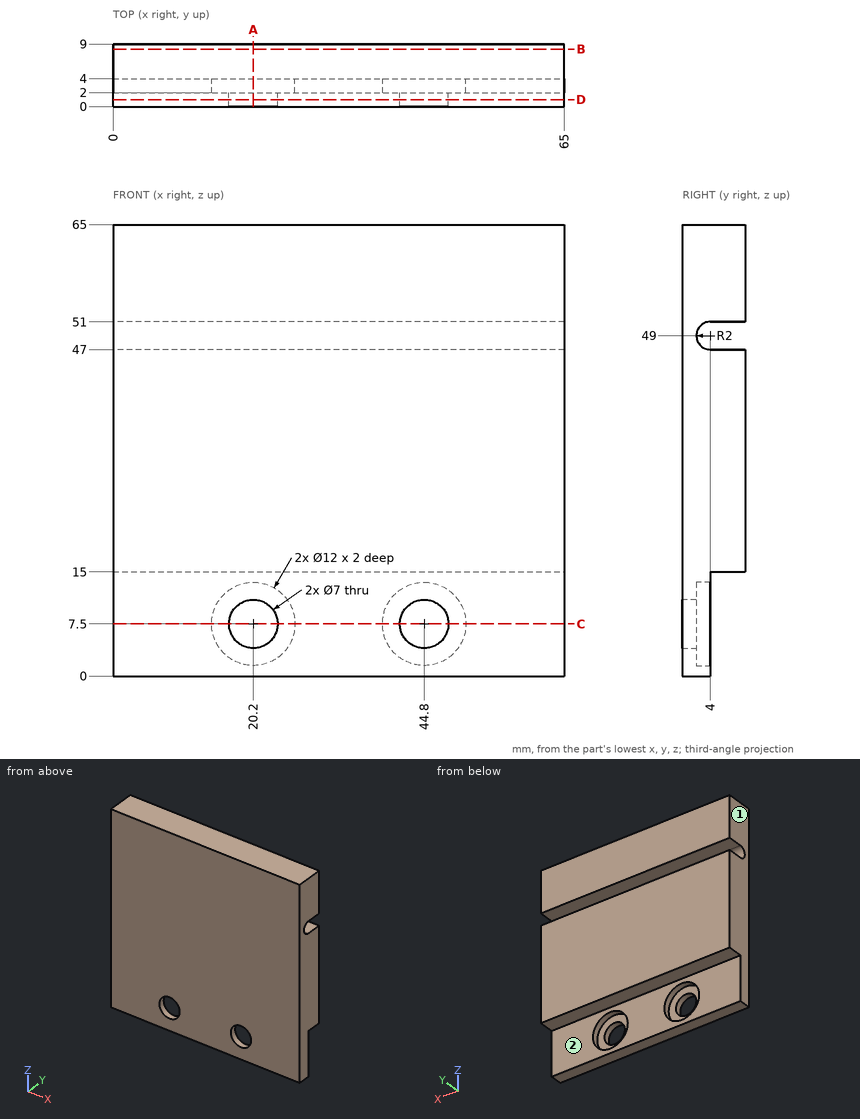
Geometry: see drawing. Coordinates: mm, zero at the bounding-box minimum. A direction names the side the tool comes from. Round coordinates to 2 decimals unless told otherwise and drop trailing zeros. Write each loop counter-clockwise with the first axis right and the second up, starting at its lowest first coordinate (ties: lowest second). Pieces come first, ordered by that corner, then holes.
1) Cut plane A-A (x = 20.2). Return the cut outline in (y, z), then the cut area to 3 significant figures.
2) Contact query for flat-ended pins moving along their axis: P1, Ø1.5, axis at x = 42, y = 7.5, coming from the -Z side; P2, Ø11, axis at x = 20.2, z = 7.5, coming from the +Y side; P3, Ø13, axis at x = 47, z = 7.5, coming from the +Y side. Output: stop coordinate, or through.
3) Cut plane B-B (y = 8.25). Return the cut outline in (x, z), then the cut area to 3 significant figures.
4) Cut plane C-C (z = 7.5). Return the cut outline in (x, y).
5) Ray query, L1, parallel to X at y = 0.55, z = 7.5; L2, parallel to Z at x = 58, y = 6.5; L3, parallel to X at y = 3.5, z = 7. Return the intervals inside material, ascending.
6) Reachability of the marked faces 1 and 2 from +Z, -Z, +X, -X, +Y, -Y: full face, straight path, thin tool, end or side. Return the list, or none.
7) Cut plane D-D (y = 1). Return the cut outline in (x, z).
Geometry says:
1. outline: (0, 0) - (4, 0) - (4, 1.5) - (2, 1.5) - (2, 4) - (0, 4) - close; (0, 11) - (2, 11) - (2, 13.5) - (4, 13.5) - (4, 15) - (9, 15) - (9, 47) - (4, 47) arc R2 cw to (4, 51) - (9, 51) - (9, 65) - (0, 65) - close
1. area: 446 mm2
2. P1: stops at z = 15
2. P2: stops at y = 2
2. P3: stops at y = 4
3. outline: (0, 15) - (65, 15) - (65, 47) - (0, 47) - close; (0, 51) - (65, 51) - (65, 65) - (0, 65) - close
3. area: 2,990 mm2
4. outline: (0, 0) - (16.7, 0) - (16.7, 2) - (14.2, 2) - (14.2, 4) - (0, 4) - close; (23.7, 0) - (41.3, 0) - (41.3, 2) - (38.8, 2) - (38.8, 4) - (26.2, 4) - (26.2, 2) - (23.7, 2) - close; (48.3, 0) - (65, 0) - (65, 4) - (50.8, 4) - (50.8, 2) - (48.3, 2) - close
5. L1: x = 0 to 16.7, 23.7 to 41.3, 48.3 to 65
5. L2: z = 15 to 47, 51 to 65
5. L3: x = 0 to 14.22, 26.18 to 38.82, 50.78 to 65
6. face 1: +Z, -Z, -X, +Y, -Y
6. face 2: -Z, +X, -X, +Y
7. outline: (0, 0) - (65, 0) - (65, 65) - (0, 65) - close; hole circle Ø7 at (20.2, 7.5); hole circle Ø7 at (44.8, 7.5)
